Part print with two shaded views. Sizes in mm from the minimum x, y, z corner. Round coordinates to 2 decimals unless told otherwise and drop trailing zeros. Order: outer loops, then holes, each group sorted by start corner. A loop starts at its lowest first (then second) coordinate and runs counter-clockwise, first axis right, second up. Notation, with made-up numbers: (71, 19.25) -> (89, 19.25) arc R37 ccw to (89, 57.25) -> close; hole circle Ø7 at (-34, 22.5). An arc over 180 degrees is marked (long way). Put each result on its own line as item: value. Start each with the question number.
Q1. Cut at C-C, the plane z = 0.5. List the corners of the cut face in (x, y) (1 decimal), and give its area (3 significant figures).
Q2. Cut at B-B, the plane y = 28.5. List the corners of the cut face in (x, z) (1 decimal).
Q3. Probe L1, parallel to X at y = 7, z = 3.05 (1 decimal); L2, parallel to X at y = 39, z = 2.85 (1 decimal); L3, parallel to Y at x = 29, z = 1.75. List the from-to ranges inside material, lowest first.
Q4. Cut at A-A, the plane x = 29.5. List the corners of the cut face in (y, z) (1 decimal).
Q5. Flat gauge pins, fed straight in: P1, Ø1, axis at x = 7.5, y = 35, coming from the -Z side; P2, Ø4, axis at x = 20.91, y = 6.89, coming from the +Z side; P3, Ø1.6, axis at x = 1, z = 2, coming from the -Y side; P4, Ø1.6, axis at y = 7, z = 1.5, coming from the -X side (3 decimals). Where does each tip first touch, or does it go through?
Q6. Cut at D-D, the plane x = 21.5. List the corners of the cut face in (y, z) (1 decimal), and give its area (3 significant figures).
Q7. Pull direction X, two halves, no side cores. Call the marked faces 1 and 2: released by +X, released by -X, zero draft, split by the parting line, or undercut.
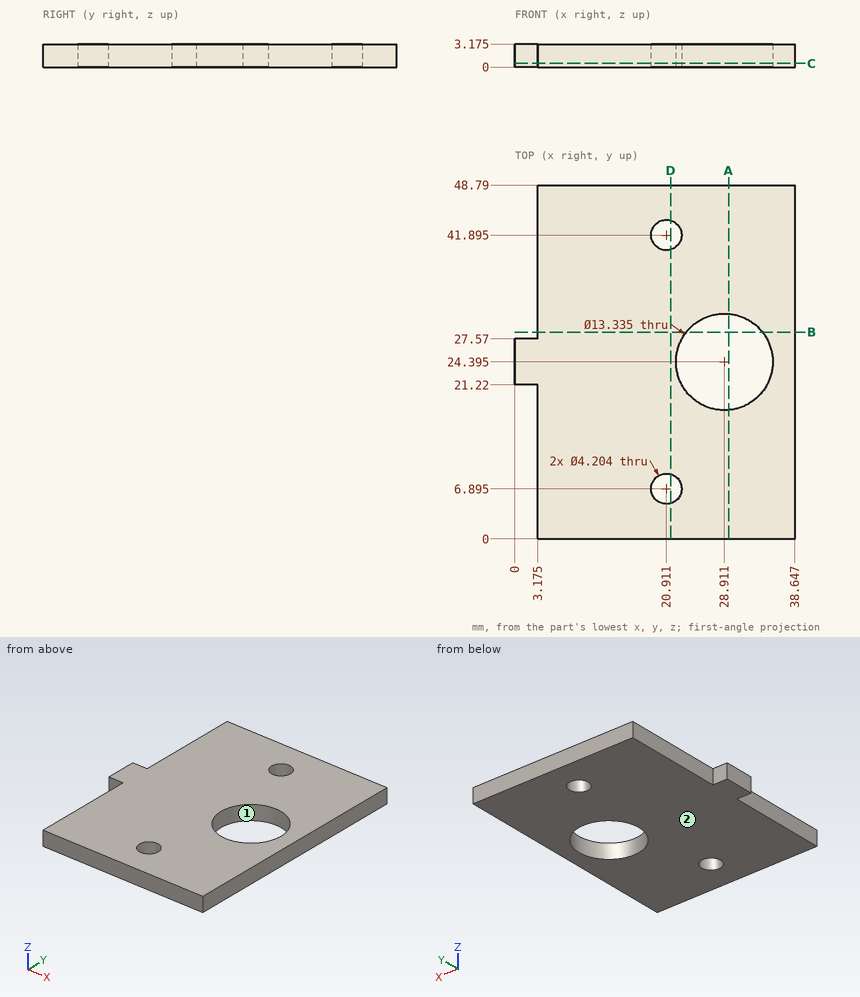
Ans:
1. outline: (0, 21.2) -> (3.2, 21.2) -> (3.2, 0) -> (38.6, 0) -> (38.6, 48.8) -> (3.2, 48.8) -> (3.2, 27.6) -> (0, 27.6) -> close; hole circle Ø4.2 at (20.9, 6.9); hole circle Ø4.2 at (20.9, 41.9); hole circle Ø13.3 at (28.9, 24.4)
1. area: 1,580 mm^2
2. outline: (3.2, 0) -> (23.7, 0) -> (23.7, 3.2) -> (3.2, 3.2) -> close; (34.2, 0) -> (38.6, 0) -> (38.6, 3.2) -> (34.2, 3.2) -> close
3. L1: x = 3.2 to 18.8, 23 to 38.6
3. L2: x = 3.2 to 38.6
3. L3: y = 0 to 17.73, 31.06 to 48.79
4. outline: (0, 0) -> (17.8, 0) -> (17.8, 3.2) -> (0, 3.2) -> close; (31, 0) -> (48.8, 0) -> (48.8, 3.2) -> (31, 3.2) -> close
5. P1: stops at z = 0
5. P2: passes through
5. P3: stops at y = 21.22
5. P4: stops at x = 3.175
6. outline: (0, 0) -> (4.9, 0) -> (4.9, 3.2) -> (0, 3.2) -> close; (8.9, 0) -> (39.9, 0) -> (39.9, 3.2) -> (8.9, 3.2) -> close; (43.9, 0) -> (48.8, 0) -> (48.8, 3.2) -> (43.9, 3.2) -> close
6. area: 129 mm^2
7. face 1: undercut
7. face 2: zero draft
